Part model, mm, in its own coordinate system. A direction names the side the tool comes from. Give positions to 0.01 mm unless a question says otherwise; leave off trailing zeros. Order: outer loops, then holes, each group sorted by start corner. A loop starts at its lowest first (then second) coordinate and runs counter-clockwise, first axis right, second up.
Autodesk Inventor part; units mm, degrees
ref_plane "YZ Plane" through (0, 0, 0) normal (1, 0, 0) x (0, 1, 0)
ref_plane "XZ Plane" through (0, 0, 0) normal (0, 1, 0) x (-1, 0, 0)
ref_plane "XY Plane" through (0, 0, 0) normal (0, 0, 1) x (1, 0, 0)
sketch "Sketch1" plane through (0, 0, 0) normal (1, 0, 0) x (0, 1, 0)
  line L0 (0, 0) -> (101.6, 0)
  line L1 (101.6, 0) -> (101.6, -101.6)
  line L2 (101.6, -101.6) -> (0, -101.6)
  line L3 (0, -101.6) -> (0, 0)
  dimension "d0" = 101.6
  dimension "d1" = 101.6
extrude "Extrusion1" add sketch "Sketch1" along normal blind 25.4
sketch "Sketch2" plane through (25.4, 0, 0) normal (1, 0, 0) x (0, 0, -1)
  line L0 (0, 101.6) -> (0, 0)
  line L1 (0, 0) -> (12.7, 0)
  line L2 (12.7, 0) -> (12.7, 6.35)
  line L3 (12.7, 6.35) -> (0, 6.35)
  line L4 (0, 6.35) -> (0, 0)
  line L5 (101.6, 0) -> (101.6, 101.6)
  line L6 (101.6, 0) -> (88.9, 0)
  line L7 (88.9, 0) -> (88.9, 6.35)
  line L8 (88.9, 6.35) -> (101.6, 6.35)
  line L9 (101.6, 6.35) -> (101.6, 0)
  line L10 (101.6, 101.6) -> (0, 101.6)
  line L11 (50.8, 101.6) -> (50.8, 76.2)
  line L12 (25.273, 58.7121) -> (76.327, 58.7121)
  line L13 (76.327, 58.7121) -> (76.327, 93.6879)
  line L14 (76.327, 93.6879) -> (25.273, 93.6879)
  line L15 (25.273, 93.6879) -> (25.273, 58.7121)
  line L16 (25.273, 58.7121) -> (76.327, 93.6879) construction
  line L17 (76.327, 58.7121) -> (25.273, 93.6879) construction
  line L18 (74.9076, 71.12) -> (101.6, 71.12)
  line L19 (101.6, 71.12) -> (101.6, 81.28)
  line L20 (101.6, 81.28) -> (74.9076, 81.28)
  line L21 (74.9076, 81.28) -> (74.9076, 71.12)
  line L22 (74.9076, 71.12) -> (101.6, 81.28) construction
  line L23 (101.6, 71.12) -> (74.9076, 81.28) construction
  line L24 (25.273, 93.6879) -> (25.273, 83.5279)
  line L25 (25.273, 58.7121) -> (25.273, 70.1421)
  line L26 (25.273, 70.1421) -> (0, 81.28)
  line L27 (25.273, 83.5279) -> (0, 95.6039)
  line L28 (0, 81.28) -> (0, 95.6039)
  line L29 (25.273, 83.5279) -> (25.273, 70.1421)
  point P0 (88.2538, 76.2)
  point P1 (76.327, 81.28)
  point P2 (76.327, 71.12)
  dimension "d4" = 12.7
  dimension "d5" = 6.35
  dimension "d6" = 12.7
  dimension "d7" = 6.35
  dimension "d8" = 25.4
  dimension "d9" = 51.054
  dimension "d10" = 34.9758
  dimension "d20" = 10.16
  dimension "d21" = 10.16
  dimension "d22" = 11.43
extrude "Extrusion2" cut sketch "Sketch2" against normal blind 25.4 contours L27 L15 L26 L0 | L15 L14 L13 L20 L21 L18 L12 | L5 L18 L13 L20 | L13 L18 L21 L20
hole "Hole1" at (25.4, 6.35, -88.9) at (25.4, 6.35, -12.7) direction (-1, 0, 0) diameter 4.9784 end through all
sketch "Sketch5" plane through (25.4, 0, 0) normal (1, 0, 0) x (0, 0, -1)
  line L0 (0, 101.6) -> (0, 95.6039)
  line L1 (25.273, 58.7121) -> (76.327, 58.7121)
  line L2 (0, 101.6) -> (25.273, 101.6)
  line L3 (25.273, 101.6) -> (25.273, 58.7121)
  line L4 (25.273, 58.7121) -> (0, 58.7121)
  line L5 (0, 58.7121) -> (0, 101.6)
  line L6 (101.6, 81.28) -> (101.6, 101.6)
  line L7 (76.327, 58.7121) -> (101.6, 58.7121)
  line L8 (101.6, 58.7121) -> (101.6, 101.6)
  line L9 (101.6, 101.6) -> (76.327, 101.6)
  line L10 (76.327, 101.6) -> (76.327, 58.7121)
  point P0 (0, 0)
extrude "Extrusion4" add sketch "Sketch5" against normal blind 3.175
sketch "Sketch6" plane through (25.4, 0, 0) normal (1, 0, 0) x (0, 0, -1)
  line L0 (76.327, 93.6879) -> (25.273, 93.6879)
  line L1 (50.8, 93.6879) -> (43.7642, 93.6879)
  line L2 (43.7642, 93.6879) -> (43.7642, 97.6503)
  line L3 (101.6, 101.6) -> (0, 101.6)
  line L4 (40.4622, 100.9523) -> (47.0662, 100.9523)
  line L5 (47.0662, 100.9523) -> (47.0662, 94.3483)
  line L6 (47.0662, 94.3483) -> (40.4622, 94.3483)
  line L7 (40.4622, 94.3483) -> (40.4622, 100.9523)
  line L8 (40.4622, 100.9523) -> (47.0662, 94.3483) construction
  line L9 (47.0662, 100.9523) -> (40.4622, 94.3483) construction
  point P0 (0, 0)
  dimension "d30" = 7.0358
  dimension "d31" = 3.9624
  dimension "d32" = 6.604
  dimension "d33" = 6.604
extrude "Extrusion5" cut sketch "Sketch6" against normal blind 25.4
sketch "Sketch7" plane through (0, 101.6, 0) normal (0, 1, 0) x (1, 0, 0)
  line L0 (25.4, 40.4622) -> (0, 40.4622)
  line L1 (25.4, 47.0662) -> (0, 47.0662)
  line L2 (0, 47.0662) -> (0, 43.7642)
  line L3 (0, 101.6) -> (0, 0)
  line L4 (0, 43.7642) -> (3.94, 43.7642)
  dimension "d36" = 3.302
  dimension "d37" = 3.94
hole "Hole2" at (3.94, 101.6, -43.7642) direction (0, -1, 0) diameter 4.318 depth 6.35 tip angle 118
sketch "Sketch8" plane through (25.4, 94.3483, -40.4622) normal (0, 1, 0) x (1, 0, 0)
  point P0 (-25.4, -40.4622)
  point P1 (-21.46, 3.302)
hole "Hole3" at (3.94, 94.3483, -43.7642) direction (0, -1, 0) diameter 2.6416 depth 10.9728 tip angle 118
properties part number "Al thermal core"
Item 1: Pull direction Y, two halves, no side cores. Call faces 1 (the face through (13, 93.688, -51)), 2 (the face through (13, 101.6, -50)), 3 (the face through (13, 84, -25.273)), 4 (the face through (13, 52, -101.6)): released by +Y, released by -Y, zero draft, split by the parting line, or undercut.
Item 2: Band-saw the part on C-C on x = 17.5. List the corners of the cut face in (y, z).
Item 3: Drill centre lines: probe 1 along Y at (x, z) = (23.75, -41.5); probe 2 along Y at (x, z) = (5.5, -88.9); probe 3 along Z at (x, y) = (8.75, 6.35). Where is each one in solid material? Low to high.
Item 4: Drop a flat-ended pin along its axis: P1, Ø10, axis at x = 5.5, y = 52, coming from the +Z side. Give the stop position or say it passes through.
Item 5: Band-saw the part on A-A on x = 3.94. Give the number of separate pieces and of enclosed holes in the cut face, plus the area to 3 significant figures.
Item 6: Band-saw the part on D-D on z = -51. List the corners of the cut face in (x, y), plus the area to 3 significant figures.
Item 7: Band-saw the part on B-B on y = 6.35. List the corners of the cut face in (x, z).
Item 8: Which spindle directions (+Z, -Z, +X, -X, +Y, -Y) get a long thin tool onto all of the face, cutting with end or side? Do faces 5 (the face through (13, 98, -47.066)), 6 (the face through (3.882, 94.013, -45.084)), 7 (the face through (22.225, 76, -89)). Say none if no direction does.
Working result:
1. face 1: undercut
1. face 2: released by +Y
1. face 3: undercut
1. face 4: zero draft
2. outline: (0, -101.6) - (71.12, -101.6) - (71.12, -76.33) - (58.71, -76.33) - (58.71, -25.27) - (70.14, -25.27) - (81.28, 0) - (0, 0) - close; (81.28, -101.6) - (101.6, -101.6) - (101.6, 0) - (95.6, 0) - (83.53, -25.27) - (93.69, -25.27) - (93.69, -76.33) - (81.28, -76.33) - close; hole circle Ø4.98 at (6.35, -88.9); hole circle Ø4.98 at (6.35, -12.7); hole (94.35, -47.07) - (100.95, -47.07) - (100.95, -40.46) - (94.35, -40.46) - close
3. probe 1: y = 0 to 58.71, 93.69 to 94.35, 100.95 to 101.6
3. probe 2: y = 0 to 3.86, 8.84 to 71.12, 81.28 to 101.6
3. probe 3: z = -101.6 to -91.39, -86.41 to -15.19, -10.21 to 0
4. P1: stops at z = 0
5. separate pieces: 3
5. enclosed holes: 2
5. area: 7,840 mm2
6. outline: (0, 0) - (25.4, 0) - (25.4, 58.71) - (0, 58.71) - close; (0, 93.69) - (25.4, 93.69) - (25.4, 101.6) - (0, 101.6) - close
6. area: 1,690 mm2
7. outline: (0, -101.6) - (25.4, -101.6) - (25.4, -91.39) - (0, -91.39) - close; (0, -86.41) - (25.4, -86.41) - (25.4, -15.19) - (0, -15.19) - close; (0, -10.21) - (25.4, -10.21) - (25.4, 0) - (0, 0) - close
8. face 5: +X, -X
8. face 6: +Y
8. face 7: -Z, -X
